Design review of the part built by this model. Coordinates are the model's own, in mm. A direction names the side the tool comes from. Coordinates: 2 decimals unless noted, no trailing zeros. Loops run counter-clockwise (first coordinate to the right, second up) from the corner with the lowest first, then second, coordinate; pieces in that order, holes last. Notation, with made-up numbers: M 62.5,40 L 67.5,40 A14 cw 67.5,50 Z; hole C 61,-21 d1. An arc over 180 degrees is marked long. Answer as a JSON object with one key per item and string values. Group by question number.
1. Consider section B-B (y = 0). State the section outline as (x, z) points.
2. Consider section A-A (z = 0). State the section outline as (x, y) points, then the cut area to 3 significant figures.
3. To check wall thickness, follow probe 1 along Y at (x, z) = (89.45, 0); probe 2 along Z at (x, y) = (99.3, -0.25); probe 3 along X at (y, z) = (1.5, -10). State the ranges of each line that lie inside material, in increasing order.
4. Insertion check: pin 1 (0.9 mm diameter, centred on y = 16.5, z = -0.5, fed in from +X); pin 2 (6 mm diameter, centred on y = 5.5, z = 5.5, fed in from +X); pin 3 (5 mm diameter, centred on x = 72, z = 8.5, fed in from -Y). Each pin has a flat end and moves straight along its axis. Give the tip position at first contact, or say it passes through.
5. Draft analysis for pull direction Y (two halves, no side actions). For faces 3 (the flat face through (103.3, 0, 0)), 4 (the cylindrical face through (89.222, -17.464, 0.325)), 5 (the cylindrical face through (97.72, -1.15, -2.77)), state which applies: +Y half, -Y half, draft (parallel to the pull), parting line (faces both ways), or undercut.
6. Machinability: for faces 1 (the flat face through (87.6, 0, 16)), 2 (the cylindrical face through (98.246, -0.042, -0.672)), which of the approach directions +Z, -Z, +X, -X, +Y, -Y give a long, thin tool a straight path to every point of the face, cutting with its end or side? Answer none if there is none.
7. Consider section C-C (y = -16). State the section outline as (x, z) points, then the cut area to 3 significant figures.
from build123d import *

# Parameters (mm, degrees)
SKETCH1_R               = 20
BOSS_EXTRUDE1_DEPTH     = 90.8
SKETCH2_R               = 11
BOSS_EXTRUDE2_DEPTH     = 1.5
SKETCH3_R               = 1.5
CUT_EXTRUDE1_DEPTH      = 3.2
SKETCH4_R               = 6.5
CUT_EXTRUDE2_DEPTH      = 5
SKETCH5_R               = 3
BOSS_EXTRUDE3_DEPTH     = 16
CUT_EXTRUDE3_DEPTH      = 10
CUT_EXTRUDE3_DEPTH_BACK = 10
SKETCH6_R               = 1.25
BOSS_EXTRUDE4_START     = 5
SKETCH7_R               = 6.5
BOSS_EXTRUDE4_DEPTH     = 5


with BuildPart() as part:
    # Sketch1 → Boss-Extrude1 (new body)
    with BuildSketch(Plane(origin=(0, 0, 0), x_dir=(0, 0, -1), z_dir=(1, 0, 0))):
        Circle(SKETCH1_R)
    extrude(amount=BOSS_EXTRUDE1_DEPTH)

    # Sketch2 → Boss-Extrude2 (add)
    with BuildSketch(Plane(origin=(90.8, 0, 0), x_dir=(0, 0, -1), z_dir=(1, 0, 0))):
        Circle(SKETCH2_R)
    extrude(amount=BOSS_EXTRUDE2_DEPTH)

    # Sketch3 → Cut-Extrude1 (cut)
    with BuildSketch(Plane(origin=(90.8, 0, 0), x_dir=(0, 0, -1), z_dir=(1, 0, 0))):
        with Locations((0, 16)):
            Circle(SKETCH3_R)
        with Locations((16, 0)):
            Circle(SKETCH3_R)
        with Locations((0, -16)):
            Circle(SKETCH3_R)
        with Locations((-16, 0)):
            Circle(SKETCH3_R)
    extrude(amount=-CUT_EXTRUDE1_DEPTH, mode=Mode.SUBTRACT)

    # Sketch4 → Cut-Extrude2 (cut)
    with BuildSketch(Plane(origin=(92.3, 0, 0), x_dir=(0, 0, -1), z_dir=(1, 0, 0))):
        Circle(SKETCH4_R)
    extrude(amount=-CUT_EXTRUDE2_DEPTH, mode=Mode.SUBTRACT)

    # Sketch5 → Boss-Extrude3 (add)
    with BuildSketch(Plane(origin=(87.3, 0, 0), x_dir=(0, 0, -1), z_dir=(1, 0, 0))):
        Circle(SKETCH5_R)
    extrude(amount=BOSS_EXTRUDE3_DEPTH)

    # Sketch6 → Cut-Extrude3 (cut, two sides: drawn at the far end of the back side and taken through both)
    with BuildSketch(Plane(origin=(0, 0, 0), x_dir=(1, 0, 0), z_dir=(0, 1, 0)).offset(-CUT_EXTRUDE3_DEPTH_BACK)):
        with Locations(Location((99.3, 0, 0), (0, 0, 90))):
            Circle(SKETCH6_R)
    extrude(amount=CUT_EXTRUDE3_DEPTH + CUT_EXTRUDE3_DEPTH_BACK, mode=Mode.SUBTRACT)

    # Sketch7 → Boss-Extrude4 (add)
    with BuildSketch(Plane(origin=(87.3, 0, 0), x_dir=(0, 0, -1), z_dir=(1, 0, 0)).offset(BOSS_EXTRUDE4_START)):
        Circle(SKETCH7_R)
    extrude(amount=-BOSS_EXTRUDE4_DEPTH)


solid = part.part
Findings below:
{
 "1": {"outline": "M 0,-20 L 90.8,-20 L 90.8,-17.5 L 87.6,-17.5 L 87.6,-14.5 L 90.8,-14.5 L 90.8,-11 L 92.3,-11 L 92.3,-3 L 103.3,-3 L 103.3,3 L 92.3,3 L 92.3,11 L 90.8,11 L 90.8,14.5 L 87.6,14.5 L 87.6,17.5 L 90.8,17.5 L 90.8,20 L 0,20 Z; hole C 99.3,0 d2.5"},
 "2": {"outline": "M 0,-20 L 90.8,-20 L 90.8,-17.5 L 87.6,-17.5 L 87.6,-14.5 L 90.8,-14.5 L 90.8,-11 L 92.3,-11 L 92.3,-3 L 98.05,-3 L 98.05,3 L 92.3,3 L 92.3,11 L 90.8,11 L 90.8,14.5 L 87.6,14.5 L 87.6,17.5 L 90.8,17.5 L 90.8,20 L 0,20 Z; M 100.55,-3 L 103.3,-3 L 103.3,3 L 100.55,3 Z", "area": "3,700 mm^2"},
 "3": {"probe 1": "y = -20 to -17.5, -14.5 to 14.5, 17.5 to 20", "probe 2": "z = -2.99 to -1.25, 1.25 to 2.99", "probe 3": "x = 0 to 92.3"},
 "4": {"pin 1": "stops at x = 87.6", "pin 2": "stops at x = 92.3", "pin 3": "stops at y = -19.08"},
 "5": {"face 3": "draft", "face 4": "undercut", "face 5": "parting line"},
 "6": {"face 1": "+X", "face 2": "+Y, -Y"},
 "7": {"outline": "M 0,-12 L 90.8,-12 L 90.8,-1.5 L 87.6,-1.5 L 87.6,1.5 L 90.8,1.5 L 90.8,12 L 0,12 Z", "area": "2,170 mm^2"}
}
